Answer from the drawing. Dimensions are ordinates in mm from the lowest x, y and z of the part. A direction names the side the tool comes from. Give positions to 0.01 mm unless a question says otherwise; leave off trailing zeros. Loops run counter-clockwise (first coordinate to the right, second up) from the corner with the lowest first, then second, coordinate; pieces in that order, holes last.
Item 1: Each of these flat-tipped pins is pushed along its axis until it touches: pin 1 Ø5.5 at (x, z) = (5, 30) entering from +Y; pin 2 Ø2 at (y, z) = (8, 23.5) entering from -X; pin 3 Ø2 at (x, z) = (5, 5) entering from -Y. Where does it stop, or does it pass through?
Item 2: Consider line 1 along Z through (x, y) = (30, 4); line 2 along Z through (x, y) = (17.5, 17). Determine where each line is inside the solid, lowest interval first.
Item 3: Section B-B, the plane y = 14 is taken. Give the vertices of the cut face in (x, z).
Item 4: Section C-C, the plane z = 2.5 is taken. Give the vertices of the cut face in (x, y).
Item 5: Section A-A, the plane y = 7.5 is taken. Give the vertices of the cut face in (x, z), and give its area (3 significant figures).
Item 6: The mould has two halves that part along X. Classify the marked faces 1, 2 and 3: pulls with the +X half, pulls with the -X half, needs draft (parallel to the pull), parting line crosses it, or undercut.
Item 7: A tool of negligible diameter and unlimited length cuts with its end or side. For the marked faces 4 and 5, from which of +Z, -Z, +X, -X, +Y, -Y can it reach the whole face along a straight path? Write none if from no direction.
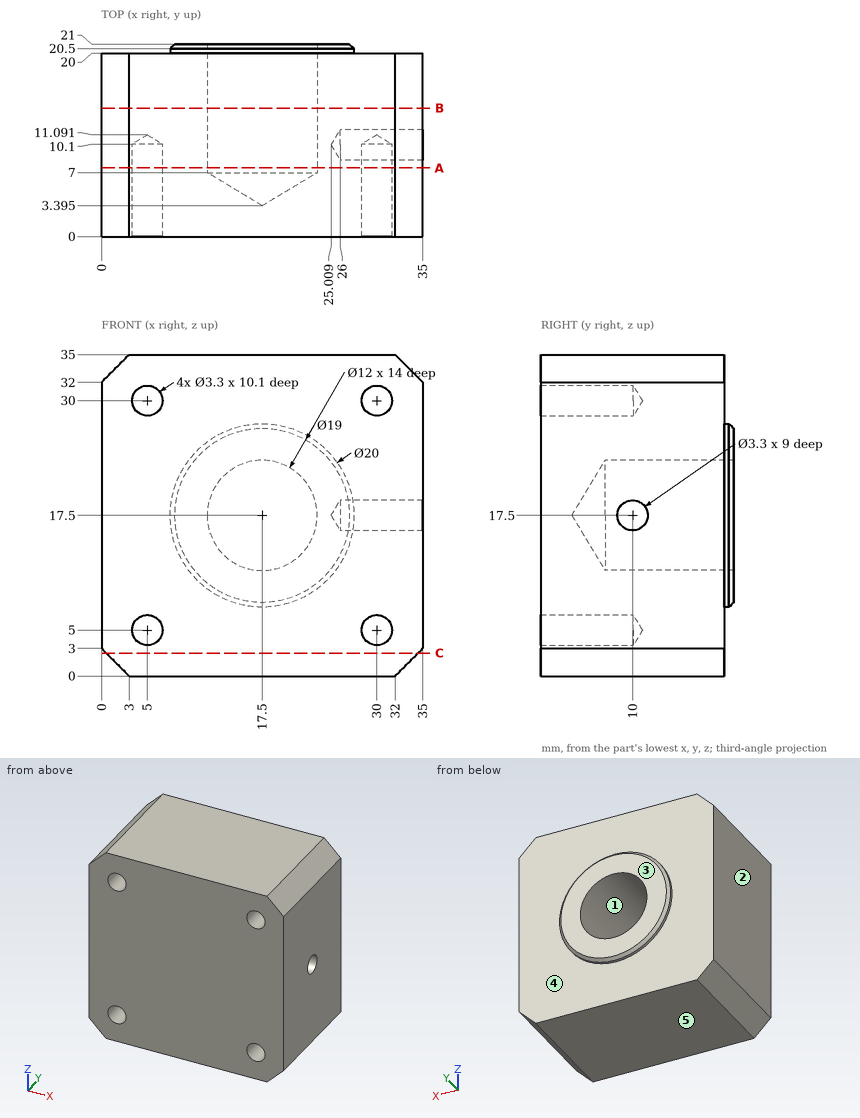
Worked answers:
1. pin 1: stops at y = 20
1. pin 2: stops at x = 0
1. pin 3: stops at y = 10.49
2. line 1: z = 0 to 3.35, 6.65 to 28.35, 31.65 to 35
2. line 2: z = 0 to 11.5, 23.5 to 35
3. outline: (0, 3) - (3, 0) - (32, 0) - (35, 3) - (35, 32) - (32, 35) - (3, 35) - (0, 32) - close; hole circle Ø12 at (17.5, 17.5)
4. outline: (0.5, 0) - (34.5, 0) - (34.5, 20) - (0.5, 20) - close
5. outline: (0, 3) - (3, 0) - (32, 0) - (35, 3) - (35, 32) - (32, 35) - (3, 35) - (0, 32) - close; hole circle Ø3.3 at (5, 5); hole circle Ø3.3 at (5, 30); hole circle Ø12 at (17.5, 17.5); hole circle Ø3.3 at (30, 5); hole circle Ø3.3 at (30, 30)
5. area: 1,060 mm2
6. face 1: undercut
6. face 2: pulls with the -X half
6. face 3: needs draft
7. face 4: +Y
7. face 5: -Z, +X, -X, +Y, -Y
